For this review, take the finished solid that the model builds, in its own axes (mm). A direction names the side the tool comes from. Give positions to 0.01 mm unless a question says otherwise; leave off trailing zeros. Order: outer loops, then holes, each group sorted by start corner. A loop starts at its lowest first (then second) coordinate and runs counter-clockwise, first axis right, second up. Notation, with made-up numbers: M -23,79 L -13,79 A20 cw -13,112 Z; hole C 5,51.25 d5. An arc over 180 degrees is marked long. Use CSV: the item, a comma, the result in double quotes. Start each with the question number.
(1) Tool access review of faces 4 (the face through (-1.5, 22.81, 0.07)), 5 (the face through (1.617, 2.958, -0.67)), 6 (the face through (2.6, 9.9, -1.5)): name each direction out of +Z, -Z, +X, -X, +Y, -Y from which nothing blocks a thin tool from reaching the whole face with its end or side.
(2) Consider section C-C (y = 11.5). Write out the cut boundary in (x, z), and give its area (3 significant figures).
(3) Clearance check with flat-ended pins moving along their axes: P1, Ø3, axis at y = 15.5, z = -2, coming from the -X side; P2, Ø3, axis at x = 0, z = 0, coming from the -Y side. State where each tip first meets the part, or that it passes through.
(4) Consider section D-D (z = -2.2). Write out the cut boundary in (x, y), and give its area (3 significant figures).
(5) Wall thickness on L1, parallel to Z at x = 0, y = 3.9; L2, parallel to Y at x = -0.25, z = 1.35; L3, parallel to Y at x = -2.25, z = -1.7: over which ranges is each line inside the solid? List them lowest first. Write a range as from..to.
(6) Consider section B-B (z = 0.4). Write out the cut boundary in (x, y), and give its area (3 significant figures).
(7) Consider section A-A (x = 0). Write out the cut boundary in (y, z), and give its area (3 significant figures).
(8) Draft analysis for pull direction X (two halves, no side actions). For faces 1 (the face through (-2.6, 9.9, 1.5)), 2 (the face through (0, 6, 0)), 3 (the face through (0, 10, 3)), state which applies: pulls with the +X half, pulls with the -X half, needs draft (parallel to the pull), parting line crosses it, or undercut.
Autodesk Inventor part; units mm, degrees
ref_plane "YZ Plane" through (0, 0, 0) normal (1, 0, 0) x (0, 1, 0)
ref_plane "XZ Plane" through (0, 0, 0) normal (0, 1, 0) x (-1, 0, 0)
ref_plane "XY Plane" through (0, 0, 0) normal (0, 0, 1) x (1, 0, 0)
sketch "Sketch1" plane through (0, 0, 0) normal (0, 1, 0) x (-1, 0, 0)
  line L0 (-3.4641, 0) -> (-1.7321, 3)
  line L1 (-1.7321, 3) -> (1.7321, 3)
  line L2 (1.7321, 3) -> (3.4641, 0)
  line L3 (3.4641, 0) -> (1.7321, -3)
  line L4 (1.7321, -3) -> (-1.7321, -3)
  line L5 (-1.7321, -3) -> (-3.4641, 0)
  point P0 (0, 0)
  point P1 (0, 0)
  dimension "d1" = 6
extrude "Extrusion1" add sketch "Sketch1" along normal blind 20
sketch "Sketch2" plane through (0, 0, 0) normal (0, -1, 0) x (1, 0, 0)
  circle A0 centre (0, 0) radius 1.75
  dimension "d4" = 3.5
sketch "Sketch3" plane through (0, 20, 0) normal (0, 1, 0) x (1, 0, 0)
  circle A0 centre (0, 0) radius 1.5
  dimension "d5" = 3
extrude "Extrusion2" add sketch "Sketch3" along normal blind 5.7
extrude "Extrusion3" cut sketch "Sketch2" against normal blind 6
thread "Thread1"
thread "Thread2"
properties part number "spacer2cm"
Check result:
1,face 4,"+Y"
1,face 5,"-Y"
1,face 6,"-Z, +X, +Y, -Y"
2,outline,"M -3.46,0 L -1.73,-3 L 1.73,-3 L 3.46,0 L 1.73,3 L -1.73,3 Z"
2,area,"31.2 mm^2"
3,P1,"stops at x = -3.18"
3,P2,"stops at y = 6"
4,outline,"M -2.19,0 L 2.19,0 L 2.19,20 L -2.19,20 Z"
4,area,"87.8 mm^2"
5,L1,"z = -3..-1.75, 1.75..3"
5,L2,"y = 6..25.7"
5,L3,"y = 0..20"
6,outline,"M -3.23,0 L -1.7,0 L -1.7,6 L 1.7,6 L 1.7,0 L 3.23,0 L 3.23,20 L 1.45,20 L 1.45,25.7 L -1.45,25.7 L -1.45,20 L -3.23,20 Z"
6,area,"125 mm^2"
7,outline,"M 0,-3 L 20,-3 L 20,-1.5 L 25.7,-1.5 L 25.7,1.5 L 20,1.5 L 20,3 L 0,3 L 0,1.75 L 6,1.75 L 6,-1.75 L 0,-1.75 Z"
7,area,"116 mm^2"
8,face 1,"pulls with the -X half"
8,face 2,"undercut"
8,face 3,"needs draft"
